```python
from build123d import *

# Parameters (mm, degrees)
SKETCH1_R           = 3.25
BOSS_EXTRUDE1_DEPTH = 6.35


with BuildPart() as part:
    # Sketch1 → Boss-Extrude1 (new body)
    with BuildSketch(Plane.XY.offset(6.35)):
        with BuildLine():
            Line((200, 8), (0, 8))
            ThreePointArc((0, 8), (-8, 0), (0, -8))
            Line((0, -8), (200, -8))
            ThreePointArc((200, -8), (208, 0), (200, 8))
        make_face()
        with Locations((200, 0)):
            Circle(SKETCH1_R, mode=Mode.SUBTRACT)
        Circle(SKETCH1_R, mode=Mode.SUBTRACT)
        with BuildLine():
            Line((104.75, 4), (142.160898385, 4))
            ThreePointArc((142.160898385, 4), (146.160898385, 0), (142.160898385, -4))
            Line((142.160898385, -4), (104.75, -4))
            ThreePointArc((104.75, -4), (100.75, 0), (104.75, 4))
        make_face(mode=Mode.SUBTRACT)
        with BuildLine():
            Line((12, 4), (48.339101615, 4))
            ThreePointArc((48.339101615, 4), (52.339101615, 0), (48.339101615, -4))
            Line((48.339101615, -4), (12, -4))
            ThreePointArc((12, -4), (8, 0), (12, 4))
        make_face(mode=Mode.SUBTRACT)
        with BuildLine():
            Line((57.839101615, 4), (95.25, 4))
            ThreePointArc((95.25, 4), (99.25, 0), (95.25, -4))
            Line((95.25, -4), (57.839101615, -4))
            ThreePointArc((57.839101615, -4), (53.839101615, 0), (57.839101615, 4))
        make_face(mode=Mode.SUBTRACT)
        with BuildLine():
            Line((188, -4), (151.660898385, -4))
            ThreePointArc((151.660898385, -4), (147.660898385, 0), (151.660898385, 4))
            Line((151.660898385, 4), (188, 4))
            ThreePointArc((188, 4), (192, 0), (188, -4))
        make_face(mode=Mode.SUBTRACT)
    extrude(amount=-BOSS_EXTRUDE1_DEPTH)


solid = part.part
```
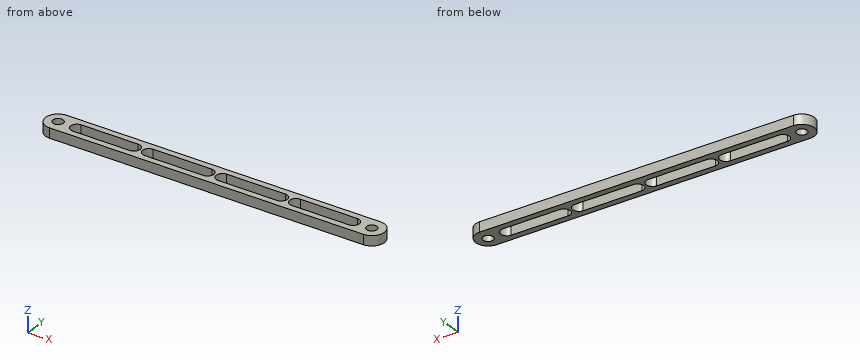
The listing builds one solid part. Answer for the finished solid, in the listing's coordinates (mm). Coordinates: 2 decimals unless noted, no trailing zeros. Write each loop counter-clockwise with the first axis right and the second up, starting at its lowest first coordinate (ties: lowest second). Pieces come first, ordered by that corner, then holes. Notation, with made-up numbers: M 20,70.5 L 63,70.5 A36 cw 63,105.5 Z; hole C 60,-10 d7. An arc over 180 degrees is marked long. Use a Markdown table: item, result. Add a question column.
1. Given P1, Ø3, axis at y = 4, z = 4, coming from the -X side; P2, Ø6, axis at x = 0, y = 0, coming from the +Z side, each flat-ended and moving along its own axis, determine where each tip first touches the part or whether it passes through.
2. Section B-B (z = 2.75) is taken. Give the vertices of the cut face in (x, y), plus the area to 3 significant figures.
3. Straight lines are drawn through the part: line 1 along Y through (x, z) = (14, 0.5); line 2 along Y through (x, z) = (0, 2); line 3 along X through (y, z) = (5.25, 3). For each, find the intervals that lie inside material, in ascending order. Write a range as [from, to].
4. Section A-A (y = 0) is taken. Give the vertices of the cut face in (x, z), plus the area to 3 significant figures.
5. Section C-C (x = 42) is taken. Give the vertices of the cut face in (y, z).
Data:
| question | item | result |
|---|---|---|
| 1 | P1 | stops at x = -7.6 |
| 1 | P2 | passes through |
| 2 | outline | M 0,-8 L 200,-8 A8 ccw 200,8 L 0,8 A8 ccw Z; hole C 0,0 d6.5; hole M 12,-4 L 48.34,-4 A4 ccw 48.34,4 L 12,4 A4 ccw Z; hole M 57.84,-4 L 95.25,-4 A4 ccw 95.25,4 L 57.84,4 A4 ccw Z; hole M 104.75,-4 L 142.16,-4 A4 ccw 142.16,4 L 104.75,4 A4 ccw Z; hole M 151.66,-4 L 188,-4 A4 ccw 188,4 L 151.66,4 A4 ccw Z; hole C 200,0 d6.5 |
| 2 | area | 1,950 mm2 |
| 3 | line 1 | y = [-8, -4], [4, 8] |
| 3 | line 2 | y = [-8, -3.25], [3.25, 8] |
| 3 | line 3 | x = [-6.04, 206.04] |
| 4 | outline | M -8,0 L -3.25,0 L -3.25,6.35 L -8,6.35 Z; M 3.25,0 L 8,0 L 8,6.35 L 3.25,6.35 Z; M 52.34,0 L 53.84,0 L 53.84,6.35 L 52.34,6.35 Z; M 99.25,0 L 100.75,0 L 100.75,6.35 L 99.25,6.35 Z; M 146.16,0 L 147.66,0 L 147.66,6.35 L 146.16,6.35 Z; M 192,0 L 196.75,0 L 196.75,6.35 L 192,6.35 Z; M 203.25,0 L 208,0 L 208,6.35 L 203.25,6.35 Z |
| 4 | area | 149 mm2 |
| 5 | outline | M -8,0 L -4,0 L -4,6.35 L -8,6.35 Z; M 4,0 L 8,0 L 8,6.35 L 4,6.35 Z |
